```python
from build123d import *

# Parameters (mm, degrees)
F0_W     = 7
F0_H     = 3.5
F1_DEPTH = 2
F0_W_2   = 12
F0_H_2   = 5
F2_DEPTH = 7.5
F4_DEPTH = 2.5
F0_W_3   = 2.1
F5_DEPTH = 4


with BuildPart() as f1:
    # F0 (on Top) → F1 (new body)
    with BuildSketch(Plane.XY):
        with Locations((-1.05, 0)):
            Rectangle(F0_W, F0_H)
    extrude(amount=F1_DEPTH)

    # F0 (on Top) → F2 (join)
    with BuildSketch(Plane.XY):
        Rectangle(F0_W_2, F0_H_2)
        Polygon((2.45, 1.75), (4.55, 1.75), (4.55, -1.75), (2.45, -1.75), (-4.55, -1.75), (-4.55, 1.75), align=None, mode=Mode.SUBTRACT)
    extrude(amount=F2_DEPTH)

    # F3 (on Front) → F4 (join, symmetric)
    with BuildSketch(Plane.XZ):
        Polygon((6, 0), (-6, 0), (6, -1.5), align=None)
    extrude(amount=F4_DEPTH, both=True)

    # F0 (on Top) → F5 (join)
    with BuildSketch(Plane.XY):
        with Locations((3.5, 0)):
            Rectangle(F0_W_3, F0_H)
    extrude(amount=F5_DEPTH)


solid = f1.part
```
CAD build for the part. Positions are in the model's coordinates, mm. A direction names the side the tool comes from. Round coordinates to 2 decimals unless told otherwise and drop trailing zeros. Write each loop counter-clockwise with the first axis right and the second up, starting at its lowest first coordinate (ties: lowest second). Pieces come first, ordered by that corner, then holes. Notation, with made-up numbers: (75.5, 86.25) - (126.5, 86.25) arc R27 cw to (126.5, 113.25) - close; hole circle Ø10 at (36.5, -11.5). An arc over 180 degrees is marked (long way). Return JSON: item names as keys, results as strings. Group by question number.
Item 1: Band-saw the part on C-C on y = 0.05. List the corners of the cut face in (x, z), plus the area to 4 significant figures.
Item 2: Flat gauge pins, fed straight in: pin 1 Ø1.5 at (x, y) = (-2.5, 1) entering from -Z; pin 2 Ø0.6 at (x, y) = (3, -0.5) entering from +Z; pin 3 Ø1.8 at (x, y) = (-1.5, 0) entering from +Z. Where does each tip first touch, or does it go through?
Item 3: Band-saw the part on A-A on z = 6.5. List the corners of the cut face in (x, y), plus the area to 4 significant figures.
Item 4: Probe probe 1 along Y at (x, z) = (-0.5, 4.75); probe 2 along X at (y, z) = (1.4, 3.25); probe 3 along X at (y, z) = (-0.75, 5.5). List the from-to ranges inside material, lowest first.
Item 5: 3-axis set-ups, long thin cutter, end or side, ignore diameter. For faces 4 (the face through (0, 1.75, 5)), 5 (the face through (0, 2.5, 3)): which of +Z, -Z, +X, -X, +Y, -Y reach the whole face in a straight line?
Item 6: Band-saw the part on B-B on x = -2. List the corners of the cut face in (y, z).
Item 7: Mould opens along X. For faces 1 (the face through (-6, 0, 4)), 2 (the face through (0, -2, 7.5)), 3 (the face through (-4.55, 0, 5)) say: +X half, -X half, draft (parallel to the pull), parting line (faces both ways), or undercut.
Item 8: Band-saw the part on D-D on z = 3.25. List the corners of the cut face in (x, y), plus the area to 3 significant figures.
Resolved:
{
 "1": {"outline": "(-6, 0) - (6, -1.5) - (6, 7.5) - (4.55, 7.5) - (4.55, 4) - (2.45, 4) - (2.45, 2) - (-4.55, 2) - (-4.55, 7.5) - (-6, 7.5) - close", "area": "53.15 mm²"},
 "2": {"pin 1": "stops at z = -0.53", "pin 2": "stops at z = 4", "pin 3": "stops at z = 2"},
 "3": {"outline": "(-6, -2.5) - (6, -2.5) - (6, 2.5) - (-6, 2.5) - close; hole (-4.55, -1.75) - (4.55, -1.75) - (4.55, 1.75) - (-4.55, 1.75) - close", "area": "28.15 mm²"},
 "4": {"probe 1": "y = -2.5 to -1.75, 1.75 to 2.5", "probe 2": "x = -6 to -4.55, 2.45 to 6", "probe 3": "x = -6 to -4.55, 4.55 to 6"},
 "5": {"face 4": "+Z", "face 5": "+Z, -Z, +X, -X, +Y"},
 "6": {"outline": "(-2.5, -0.5) - (2.5, -0.5) - (2.5, 7.5) - (1.75, 7.5) - (1.75, 2) - (-1.75, 2) - (-1.75, 7.5) - (-2.5, 7.5) - close"},
 "7": {"face 1": "-X half", "face 2": "draft", "face 3": "undercut"},
 "8": {"outline": "(-6, -2.5) - (6, -2.5) - (6, 2.5) - (-6, 2.5) - close; hole (-4.55, -1.75) - (2.45, -1.75) - (2.45, 1.75) - (-4.55, 1.75) - close", "area": "35.5 mm²"}
}
